Geometry check sheet. Reference: the model listing, model coordinates, mm. A direction names the side the tool comes from. Round coordinates to 2 decimals unless told otherwise and drop trailing zeros. Write each loop counter-clockwise with the first axis right and the second up, starting at its lowest first coordinate (ties: lowest second). Pieces come first, ordered by that corner, then holes. Notation, with made-up numbers: (19.5, 84) -> (40.5, 84) arc R4 cw to (40.5, 89) -> close; hole circle Ø3 at (48.5, -34.75). An arc over 180 degrees is marked (long way). One line per question, with ' | ' between items.
```python
from build123d import *

# Parameters (mm, degrees)
PUMP_BODY_START     = -45
SKETCH1_R           = 20
PUMP_BODY_DEPTH     = 90
MOTOR_ENDBELL_START = -45
SKETCH2_R           = 21
MOTOR_ENDBELL_DEPTH = 10
SKETCH3_W           = 54
SKETCH3_H           = 28
MOUNT_SADDLE_DEPTH  = 9
INLET_BARB_START    = -60
SKETCH4_R           = 4
INLET_BARB_DEPTH    = 15
OUTLET_BARB_START   = 45
SKETCH5_R           = 4
OUTLET_BARB_DEPTH   = 15
INLET_RIDGE_START   = -58
SKETCH6_R           = 5
INLET_RIDGE_DEPTH   = 3
OUTLET_RIDGE_START  = 55
SKETCH7_R           = 5
OUTLET_RIDGE_DEPTH  = 3
TERMINAL_POS_START  = 43
SKETCH8_W           = 3
SKETCH8_H           = 2
TERMINAL_POS_DEPTH  = 6
TERMINAL_NEG_START  = 43
SKETCH9_W           = 3
SKETCH9_H           = 2
TERMINAL_NEG_DEPTH  = 6


with BuildPart() as part:
    # Sketch1 → Pump_Body (new body)
    with BuildSketch(Plane(origin=(0, 0, 0), x_dir=(0, 0, -1), z_dir=(1, 0, 0)).offset(PUMP_BODY_START)):
        with Locations(Location((0, 25, 0), (0, 0, 180))):
            Circle(SKETCH1_R)
    extrude(amount=PUMP_BODY_DEPTH)

    # Sketch2 → Motor_EndBell (add)
    with BuildSketch(Plane(origin=(0, 0, 0), x_dir=(0, 0, -1), z_dir=(1, 0, 0)).offset(MOTOR_ENDBELL_START)):
        with Locations((0, 25)):
            Circle(SKETCH2_R)
    extrude(amount=MOTOR_ENDBELL_DEPTH)

    # Sketch3 → Mount_Saddle (add)
    with BuildSketch(Plane(origin=(0, 0, 0), x_dir=(1, 0, 0), z_dir=(0, 1, 0))):
        Rectangle(SKETCH3_W, SKETCH3_H)
    extrude(amount=MOUNT_SADDLE_DEPTH)

    # Sketch4 → Inlet_Barb (add)
    with BuildSketch(Plane(origin=(0, 0, 0), x_dir=(0, 0, -1), z_dir=(1, 0, 0)).offset(INLET_BARB_START)):
        with Locations((0, 25)):
            Circle(SKETCH4_R)
    extrude(amount=INLET_BARB_DEPTH)

    # Sketch5 → Outlet_Barb (add)
    with BuildSketch(Plane(origin=(0, 0, 0), x_dir=(0, 0, -1), z_dir=(1, 0, 0)).offset(OUTLET_BARB_START)):
        with Locations((0, 25)):
            Circle(SKETCH5_R)
    extrude(amount=OUTLET_BARB_DEPTH)

    # Sketch6 → Inlet_Ridge (add)
    with BuildSketch(Plane(origin=(0, 0, 0), x_dir=(0, 0, -1), z_dir=(1, 0, 0)).offset(INLET_RIDGE_START)):
        with Locations((0, 25)):
            Circle(SKETCH6_R)
    extrude(amount=INLET_RIDGE_DEPTH)

    # Sketch7 → Outlet_Ridge (add)
    with BuildSketch(Plane(origin=(0, 0, 0), x_dir=(0, 0, -1), z_dir=(1, 0, 0)).offset(OUTLET_RIDGE_START)):
        with Locations((0, 25)):
            Circle(SKETCH7_R)
    extrude(amount=OUTLET_RIDGE_DEPTH)

    # Sketch8 → Terminal_Pos (add)
    with BuildSketch(Plane(origin=(0, 0, 0), x_dir=(1, 0, 0), z_dir=(0, 1, 0)).offset(TERMINAL_POS_START)):
        with Locations((-27, 5)):
            Rectangle(SKETCH8_W, SKETCH8_H)
    extrude(amount=TERMINAL_POS_DEPTH)

    # Sketch9 → Terminal_Neg (add)
    with BuildSketch(Plane(origin=(0, 0, 0), x_dir=(1, 0, 0), z_dir=(0, 1, 0)).offset(TERMINAL_NEG_START)):
        with Locations((-27, -5)):
            Rectangle(SKETCH9_W, SKETCH9_H)
    extrude(amount=TERMINAL_NEG_DEPTH)


solid = part.part
```
(1) Draft check along X on faces 1 (the flat face through (-35, 17, -19)), 2 (the flat face through (27, 3, 0)), 3 (the cylindrical face through (-59.014, 28.966, 0.521)). Enter one of: +X half, -X half, draft (parallel to the pull), parting line (faces both ways), or undercut.
Resolved:
face 1: undercut | face 2: +X half | face 3: draft
(2) Access from +Z, -Z, +X, -X, +Y, -Y to the whole of each face (thin tool, end or side, straight path). Record for faces 4 (the flat face through (-27, 47, 4)), 5 (the cylindrical face through (56.48, 20.12, 1.08)), 6 (the flat face through (0, 4, -14)), 7 (the flat face through (0, 4, 14)).
Resolved:
face 4: +X, +Y | face 5: +X | face 6: -Z, +X, -X, -Y | face 7: +Z, +X, -X, -Y
(3) Sectioned sample at B-B on x = 1. Record the cut outline in (y, z).
Resolved:
outline: (0, -14) -> (9, -14) -> (9, -12) arc R20 ccw (long way) to (9, 12) -> (9, 14) -> (0, 14) -> close
(4) Go/stop test with flat-tipped pins: pin 1 (12 mm diameter, centred on y = 33.5, z = 2, fed in from +X); pin 2 (5 mm diameter, centred on y = 38.5, z = 12.5, fed in from -X); pin 3 (1 mm diameter, centred on x = 1, z = -13, fed in from +Y); pin 4 (6 mm diameter, centred on x = -30.5, y = 12.5, fed in from +Z). Record where each tip stops, or that it passes through.
Resolved:
pin 1: stops at x = 60 | pin 2: stops at x = -45 | pin 3: stops at y = 40.61 | pin 4: stops at z = 17.6
(5) Material ranges on line 1 (X direction, y = 15, z = 1.5); line 2 (Z direction, x = -28, y = 45.5); line 3 (X direction, y = 16.5, z = 19), recorded low to high.
Resolved:
line 1: x = -45 to 45 | line 2: z = -6 to -4, 4 to 6 | line 3: x = -45 to -35
(6) Sectioned sample at D-D on x = 32. Record the cut outline in (y, z).
Resolved:
outline: circle Ø40 at (25, 0)
(7) Sectioned sample at C-C on y = 31.5. Record the cut outline in (x, z).
Resolved:
outline: (-45, -19.97) -> (-35, -19.97) -> (-35, -18.91) -> (45, -18.91) -> (45, 18.91) -> (-35, 18.91) -> (-35, 19.97) -> (-45, 19.97) -> close
